```python
from build123d import *

# Parameters (mm, degrees)
SKETCH1_W           = 22.5
SKETCH1_H           = 150
SKETCH1_R           = 1
BOSS_EXTRUDE1_DEPTH = 2.3
FILLET1_R           = 11.5
THREAD1_PITCH       = 0.79375
FILLET2_R           = 1


with BuildPart() as part:
    # Sketch1 → Boss-Extrude1 (new body)
    with BuildSketch(Plane.XY):
        with Locations((0, 75)):
            Rectangle(SKETCH1_W, SKETCH1_H)
        with Locations((0, 140)):
            Circle(SKETCH1_R, mode=Mode.SUBTRACT)
        with Locations((0, 130)):
            Circle(SKETCH1_R, mode=Mode.SUBTRACT)
        with Locations((0, 120)):
            Circle(SKETCH1_R, mode=Mode.SUBTRACT)
        with Locations((0, 110)):
            Circle(SKETCH1_R, mode=Mode.SUBTRACT)
        with Locations((0, 100)):
            Circle(SKETCH1_R, mode=Mode.SUBTRACT)
    extrude(amount=BOSS_EXTRUDE1_DEPTH)

    # Fillet1
    # the kernel refuses this fillet: 11.5 mm, written as the material it takes off along each edge
    with BuildSketch(Plane(origin=(11.25, 150, -28.75), x_dir=(0, -1, 0), z_dir=(0, 0, 1)), Plane(origin=(-11.25, 150, -28.75), x_dir=(1, 0, 0), z_dir=(0, 0, 1))) as fillet1_piece_1:
        with BuildLine():
            CenterArc((FILLET1_R, -FILLET1_R), FILLET1_R, 90, 90)
            Line((0, -FILLET1_R), (0, 0))
            Line((0, 0), (FILLET1_R, 0))
        make_face()
    extrude(amount=59.8, mode=Mode.SUBTRACT)

    # Sketch3 → CSK for #6 Flat Head Machine Screw (100)1 (revolve, cut)
    with BuildSketch(Plane(origin=(0, 5.75, 0), x_dir=(0, 1, 0), z_dir=(1, 0, 0))):
        Polygon((0, 0), (0, 2.3), (1.89865, 2.3), (1.89865, 1.380025208), (3.5433, 0), align=None)
    revolve(axis=Axis((0, 5.75, -6.35), (0, 0, 1)), mode=Mode.SUBTRACT)

    # Thread1: the profile of Thread Profile1 profile screwed along a right-hand helix of 1.159023 turns, 8 arcs to a turn; built about Z, then put on its axis
    thread1_z = Axis((0, 0, 0), (0, 0, 1))
    thread1_corners = [(1.89835, 0, -0.000173205), (2.328279788, 0, 0.248046874), (2.328279788, 0, 0.347265624), (1.89835, 0, 0.595485703)]
    with BuildLine(mode=Mode.PRIVATE) as thread1_profile:
        Line(thread1_corners[0], thread1_corners[1])
        Line(thread1_corners[1], thread1_corners[2])
        Line(thread1_corners[2], thread1_corners[3])
        Line(thread1_corners[3], thread1_corners[0])
    thread1_cap = Face(thread1_profile.wire())
    thread1_turn_angles = [0, 22.5, 45, 67.5, 90, 112.5, 135, 157.5, 180, 202.5, 225, 247.5, 270, 292.5, 315, 337.5, 360]
    thread1_turn_weights = [1, 0.9238795325112867, 1, 0.9238795325112867, 1, 0.9238795325112867, 1, 0.9238795325112867, 1, 0.9238795325112867, 1, 0.9238795325112867, 1, 0.9238795325112867, 1, 0.9238795325112867, 1]
    thread1_turn_rails = [Edge.make_bspline([Vector(p[0], p[1], 0).rotate(thread1_z, thread1_turn_angles[k]) / thread1_turn_weights[k] + Vector(0, 0, p[2] + THREAD1_PITCH * thread1_turn_angles[k] / 360) for k in range(17)], [0, 0, 0, 1, 1, 2, 2, 3, 3, 4, 4, 5, 5, 6, 6, 7, 7, 8, 8, 8], 2, thread1_turn_weights) for p in thread1_corners]
    thread1_turn_sides = [Face.make_surface_from_curves(thread1_turn_rails[p[0]], thread1_turn_rails[p[1]]) for p in [(0, 1), (1, 2), (2, 3), (3, 0)]]
    thread1_last_angles = [360, 382.5, 405, 411.124204706, 417.248409411]
    thread1_last_weights = [1, 0.9238795325112867, 1, 0.9942929639578035, 1]
    thread1_last_rails = [Edge.make_bspline([Vector(p[0], p[1], 0).rotate(thread1_z, thread1_last_angles[k]) / thread1_last_weights[k] + Vector(0, 0, p[2] + THREAD1_PITCH * thread1_last_angles[k] / 360) for k in range(5)], [0, 0, 0, 1, 1, 2, 2, 2], 2, thread1_last_weights) for p in thread1_corners]
    thread1_last_sides = [Face.make_surface_from_curves(thread1_last_rails[p[0]], thread1_last_rails[p[1]]) for p in [(0, 1), (1, 2), (2, 3), (3, 0)]]
    thread1 = Plane(origin=(0, 5.75, 1.380025208), x_dir=(1, 0, 0), z_dir=(0, 0, 1)) * Solid(Shell([*thread1_turn_sides, *thread1_last_sides, thread1_cap, thread1_cap.rotate(thread1_z, 417.248409411).moved(Location((0, 0, THREAD1_PITCH * 417.248409411 / 360)))]))
    add(thread1, mode=Mode.SUBTRACT)

    # Fillet2
    fillet2_edges = [part.edges().sort_by_distance(p)[0] for p in [
        (11.25, 0, 1.15),
        (-11.25, 0, 1.15),
    ]]
    fillet(fillet2_edges, radius=FILLET2_R)


solid = part.part
```
Work out the finished part from the listing and answer in its coordinate system (mm). Give positions to 0.01 mm unless a question says otherwise; leave off trailing zeros. Loops run counter-clockwise (first coordinate to the right, second up) from the corner with the lowest first, then second, coordinate; pieces in that order, holes last. Notation, with made-up numbers: (85, 38) - (136, 38) arc R26 cw to (136, 77) - close; hole circle Ø9 at (83.25, 52). An arc over 180 degrees is marked (long way). Use CSV: the item, a comma, the result in double quotes. Start each with the question number.
(1) Find the intervals of material crossed by L1, parallel to X at y = 120, z = 1.6; L2, parallel to X at y = 5.75, z = 2; L3, parallel to Y at x = -3.25, z = 0.6, in increasing order.
(2) Find section B-B, the plane x = -7. Determine the outline of the cut face in (y, z).
(3) This flat-tipped pin is pushed along its axis until it touches: pin 1 (1 mm diameter, centred on x = 1, z = 0.5, fed in from +Y). Where does it stop, or does it pass through?
(4) Find section A-A, the plane z = 0.5. Determine the outline of the cut face in (x, y), plus the area to 3 significant figures.
Results found:
1,L1,"-11.25 to -1, 1 to 11.25"
1,L2,"-11.25 to -2.29, 1.9 to 11.25"
1,L3,"0 to 149.45"
2,outline,"(0, 0) - (147.43, 0) - (147.43, 2.3) - (0, 2.3) - close"
3,pin 1,"y = 149.98"
4,outline,"(-11.25, 1) arc R1 ccw to (-10.25, 0) - (10.25, 0) arc R1 ccw to (11.25, 1) - (11.25, 138.5) arc R11.5 ccw to (0, 150) arc R11.5 ccw to (-11.25, 138.5) - close; hole circle Ø5.89 at (0, 5.75); hole circle Ø2 at (0, 100); hole circle Ø2 at (0, 110); hole circle Ø2 at (0, 120); hole circle Ø2 at (0, 130); hole circle Ø2 at (0, 140)"
4,area,"3,270 mm^2"
